from build123d import *

# Parameters (mm, degrees)
SKETCH_1_W                  = 30
SKETCH_1_H                  = 11
EXTRUDE_1_DEPTH             = 6
SKETCH_2_W                  = 16
SKETCH_2_H                  = 2
CUT_EXTRUDE_1_DEPTH         = 144
EXTRUDE_2_DEPTH             = 192
SKETCH_4_R                  = 1.75
CUT_EXTRUDE_2_DEPTH         = 144
SKETCH_5_W                  = 11
SKETCH_5_H                  = 198
CUT_EXTRUDE_3_DEPTH         = 2.5
EXTRUDE_3_REACH             = 194.664
EXTRUDE_3_DIRECTION_2_REACH = 194.664
SKETCH_7_W                  = 1.5
SKETCH_7_H                  = 198
EXTRUDE_4_DEPTH             = 10
CUT_EXTRUDE_4_DEPTH         = 40
EXTRUDE_5_DEPTH             = 2
SKETCH_10_R                 = 1.25
CUT_EXTRUDE_5_DEPTH         = 3


with BuildPart() as part:
    # 草图1 → 凸台-拉伸1 (new body)
    with BuildSketch(Plane(origin=(0, 0, 0), x_dir=(1, 0, 0), z_dir=(0, 1, 0))):
        Rectangle(SKETCH_1_W, SKETCH_1_H)
    extrude(amount=EXTRUDE_1_DEPTH)

    # 草图2 → 切除-拉伸1 (cut)
    with BuildSketch(Plane.ZY.offset(15)):
        with Locations((-5.5, 3)):
            Rectangle(SKETCH_2_W, SKETCH_2_H)
    extrude(amount=-CUT_EXTRUDE_1_DEPTH, mode=Mode.SUBTRACT)

    # 草图3 → 凸台-拉伸2 (add)
    with BuildSketch(Plane(origin=(0, 6, 0), x_dir=(1, 0, 0), z_dir=(0, 1, 0))):
        Polygon((2, 5.5), (-2, 5.5), (-2, -3.5), (-15, -3.5), (-15, -5.5), (15, -5.5), (15, -3.5), (2, -3.5), align=None)
    extrude(amount=EXTRUDE_2_DEPTH)

    # 草图4 → 切除-拉伸2 (cut)
    with BuildSketch(Plane(origin=(0, 6, 0), x_dir=(1, 0, 0), z_dir=(0, 1, 0))):
        with Locations(Location((-7.5, 2, 0), (0, 0, 270))):
            Circle(SKETCH_4_R)
        with Locations(Location((7.5, 2, 0), (0, 0, 270))):
            Circle(SKETCH_4_R)
    extrude(amount=-CUT_EXTRUDE_2_DEPTH, mode=Mode.SUBTRACT)

    # 草图5 → 切除-拉伸3 (cut)
    with BuildSketch(Plane.ZY.offset(15)):
        with Locations((0, 99)):
            Rectangle(SKETCH_5_W, SKETCH_5_H)
    extrude(amount=-CUT_EXTRUDE_3_DEPTH, mode=Mode.SUBTRACT)

    # 凸台-拉伸3: up to this face of the body (flat: up to its plane)
    extrude_3_end = Plane(part.part.faces().sort_by_distance((0.755494505, 198, 2.324175824))[0])
    # 草图6 → 凸台-拉伸3 (add, up to the picked face)
    with BuildSketch(Plane(origin=(0, 6, 0), x_dir=(1, 0, 0), z_dir=(0, 1, 0)), mode=Mode.PRIVATE) as extrude_3_sk1:
        with BuildLine():
            Line((-22.5, 7.5), (-25.5, 7.5))
            ThreePointArc((-25.5, 7.5), (-21.692388155, -1.692388155), (-12.5, -5.5))
            Line((-12.5, -5.5), (-12.5, -2.5))
            ThreePointArc((-12.5, -2.5), (-19.571067812, 0.428932188), (-22.5, 7.5))
        make_face()
    extrude_3_tool1 = split(extrude(extrude_3_sk1.sketch, amount=EXTRUDE_3_REACH, mode=Mode.PRIVATE), bisect_by=extrude_3_end, keep=Keep.BOTH, mode=Mode.PRIVATE)
    add(extrude_3_tool1.solids().sort_by(Axis((-19.862646, 6, -0.137354), (0, 1, 0)))[0])

    # 凸台-拉伸3 direction 2: up to this face of the body (flat: up to its plane)
    extrude_3_direction_2_end = Plane(part.part.faces().sort_by_distance((1.334914955, 0, 0.135863928))[0])
    # 草图6 → 凸台-拉伸3 direction 2 (add, up to the picked face)
    with BuildSketch(Plane(origin=(0, 6, 0), x_dir=(1, 0, 0), z_dir=(0, 1, 0)), mode=Mode.PRIVATE) as extrude_3_direction_2_sk1:
        with BuildLine():
            Line((-22.5, 7.5), (-25.5, 7.5))
            ThreePointArc((-25.5, 7.5), (-21.692388155, -1.692388155), (-12.5, -5.5))
            Line((-12.5, -5.5), (-12.5, -2.5))
            ThreePointArc((-12.5, -2.5), (-19.571067812, 0.428932188), (-22.5, 7.5))
        make_face()
    extrude_3_direction_2_tool1 = split(extrude(extrude_3_direction_2_sk1.sketch, amount=-EXTRUDE_3_DIRECTION_2_REACH, mode=Mode.PRIVATE), bisect_by=extrude_3_direction_2_end, keep=Keep.BOTH, mode=Mode.PRIVATE)
    add(extrude_3_direction_2_tool1.solids().sort_by(Axis((-19.862646, 6, -0.137354), (0, -1, 0)))[0])

    # 草图7 → 凸台-拉伸4 (add)
    with BuildSketch(Plane(origin=(0, 0, -7.5), x_dir=(-1, 0, 0), z_dir=(0, 0, -1))):
        with Locations((23.25, 99)):
            Rectangle(SKETCH_7_W, SKETCH_7_H)
    extrude(amount=EXTRUDE_4_DEPTH)

    # 草图8 → 切除-拉伸4 (cut)
    with BuildSketch(Plane(origin=(-12.5, 0, 0), x_dir=(0, 0, -1), z_dir=(1, 0, 0))):
        Polygon((26.892505746, 198), (-2.5, 198), (-2.5, 6), (-2.5, -9.514717226), (26.892505746, -9.514717226), align=None)
        Polygon((-3.5, 6), (-3.5, 198), (-26.700940199, 198), (-26.700940199, -9.514717226), (-2.5, -9.514717226), (-2.5, 6), align=None)
    extrude(amount=CUT_EXTRUDE_4_DEPTH, mode=Mode.SUBTRACT)


with BuildPart() as cut_extrude_4_kept_piece:
    # of the separate pieces the step leaves, the one the design keeps (cut_extrude_4_pieces_kept)
    add(part.part.solids().sort_by_distance((-22.5, 0, -7.5))[0])

    # 草图9 → 凸台-拉伸5 (add)
    with BuildSketch(Plane(origin=(0, 198, 0), x_dir=(1, 0, 0), z_dir=(0, 1, 0))):
        with BuildLine():
            Line((-12.5, -2.5), (-12.5, 7.5))
            Line((-12.5, 7.5), (-22.5, 7.5))
            ThreePointArc((-22.5, 7.5), (-19.571067812, 0.428932188), (-12.5, -2.5))
        make_face()
    extrude_5 = extrude(amount=-EXTRUDE_5_DEPTH)

    # 草图10 → 切除-拉伸5 (cut)
    with BuildSketch(Plane(origin=(0, 196, 0), x_dir=(-1, 0, 0), z_dir=(0, -1, 0))):
        with Locations(Location((14.8, 2.5, 0), (0, 0, 90))):
            Circle(SKETCH_10_R)
        with Locations(Location((17.5, 5.2, 0), (0, 0, 90))):
            Circle(SKETCH_10_R)
    cut_extrude_5 = extrude(amount=-CUT_EXTRUDE_5_DEPTH, mode=Mode.SUBTRACT)

    # 镜向2: 凸台-拉伸5, 切除-拉伸5 across plane
    add(extrude_5.mirror(Plane(origin=(0, 99, 0), x_dir=(0, 0, 1), z_dir=(0, -1, 0))))
    add(cut_extrude_5.mirror(Plane(origin=(0, 99, 0), x_dir=(0, 0, 1), z_dir=(0, -1, 0))), mode=Mode.SUBTRACT)


solid = cut_extrude_4_kept_piece.part
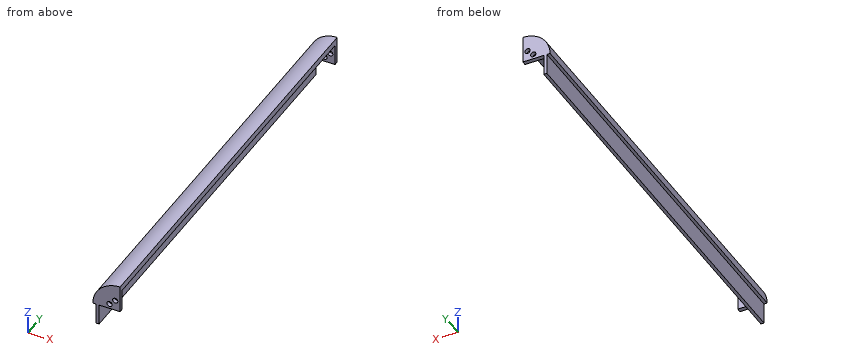
Design review of the part built by this model. Coordinates are the model's own, in mm. Round coordinates to 2 decimals unless told otherwise and drop trailing zeros. Write each loop counter-clockwise with the first axis right and the second up, starting at its lowest first coordinate (ties: lowest second). Pieces come first, ordered by that corner, then holes. Notation, with made-up numbers: M 16,-29.75 L 49,-29.75 A13 cw 49,-21.75 Z; hole C 38.25,46.25 d1. An arc over 180 degrees is marked long. One line per item, written item: value. Start each with the question number.
1. To check wall thickness, follow probe 1 along Y at (x, z) = (-18, -1.5); probe 2 along Z at (x, y) = (-17.5, 1.6); probe 3 along X at (y, z) = (196.45, -5.2). State the ranges of each line that lie inside material, in increasing order. Write a range as from..to.
2. Take a section at A-A on y = 61. State the section outline as (x, z) points, then the cut area to 3 significant figures.
3. Take a section at B-B on x = -20.5. State the section outline as (y, z) points.
4. Clearance check with flat-ended pins moving along their axes: P1, Ø2, axis at x = -17.5, y = 197.5, coming from the -Z side; P2, Ø5, axis at x = -19, z = -13, coming from the +Y side; P3, Ø2, axis at y = 161.5, z = -7, coming from the +X side; P4, Ø1.5, axis at x = -14.5, y = 79.5, coming from the +Z side. State where each tip first meets the part, or that it passes through.
Computed:
1. probe 1: y = 0..2, 196..198
1. probe 2: z = -7.5..-6.45, -3.95..4.5
1. probe 3: x = -25.29..-18.75, -16.25..-12.5
2. outline: M -25.5,-7.5 L -24,-7.5 L -24,-17.5 L -22.5,-17.5 L -22.5,-7.5 A10 cw -12.5,2.5 L -12.5,5.5 A13 ccw Z
2. area: 69.2 mm²
3. outline: M 0,-7.5 L 2,-7.5 L 2,-1.5 L 196,-1.5 L 196,-7.5 L 198,-7.5 L 198,2.75 L 0,2.75 Z
4. P1: stops at z = -7.5
4. P2: passes through
4. P3: stops at x = -22.39
4. P4: stops at z = 5.44
